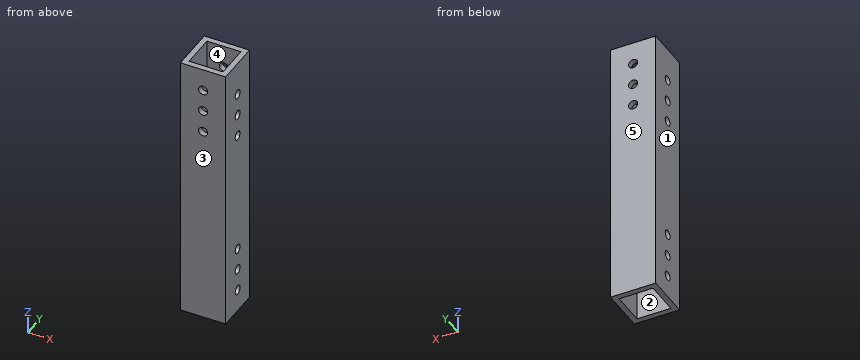
from build123d import *

# Parameters (mm, degrees)
SKETCH3_W              = 25.4
SKETCH3_H              = 25.4
SKETCH3_W_2            = 19.05
SKETCH3_H_2            = 19.05
BOSS_EXTRUDE1_DEPTH    = 152.4
F_10_CLEARANCE_HOLE1_D = 5.1054
F_10_CLEARANCE_HOLE2_D = 5.1054
F_10_CLEARANCE_HOLE3_D = 5.1054


with BuildPart() as part:
    # Sketch3 → Boss-Extrude1 (new body)
    with BuildSketch(Plane.XY):
        with Locations((-12.7, 12.7)):
            Rectangle(SKETCH3_W, SKETCH3_H)
        with Locations((-12.7, 12.7)):
            Rectangle(SKETCH3_W_2, SKETCH3_H_2, mode=Mode.SUBTRACT)
    extrude(amount=BOSS_EXTRUDE1_DEPTH)

    # #10 Clearance Hole1 (through all)
    with Locations(Plane(origin=(0, 25.4, 0), x_dir=(1, 0, 0), z_dir=(0, 1, 0))):
        with Locations((-12.7, -139.7), (-12.7, -127), (-12.7, -114.3)):
            Hole(F_10_CLEARANCE_HOLE1_D / 2)

    # #10 Clearance Hole2 (through all)
    with Locations(Plane.ZY.offset(25.4)):
        with Locations((133.35, 12.7), (120.65, 12.7), (107.95, 12.7)):
            Hole(F_10_CLEARANCE_HOLE2_D / 2)

    # #10 Clearance Hole3 (through all)
    with Locations(Plane(origin=(0, 0, 0), x_dir=(0, 0, -1), z_dir=(1, 0, 0))):
        with Locations((-12.7, 12.7), (-25.4, 12.7), (-38.1, 12.7)):
            Hole(F_10_CLEARANCE_HOLE3_D / 2)


solid = part.part
Verification items for the finished model (mm, model axes). Face numbers are marked on the shaded views. A direction names the side the tool comes from. Coordinates: 2 decimals unless noted, no trailing zeros. Loops run counter-clockwise (first coordinate to the right, second up) from the corner with the lowest first, then second, coordinate; pieces in that order, holes last. Notation, with made-up numbers: M 25.25,32 L 33.25,32 A17 cw 33.25,39 Z; hole C -5.5,41 d1. An arc over 180 degrees is marked long. One line per item, written item: value.
1. Section check B-B on y = 19. Record the cut outline in (x, z) (3 decimals), plus the area to 3 significant figures.
Answers follow:
outline: M -25.4,0 L -22.225,0 L -22.225,152.4 L -25.4,152.4 Z; M -3.175,0 L 0,0 L 0,152.4 L -3.175,152.4 Z
area: 968 mm^2
2. Section check C-C on x = -6. Record the cut outline in (y, z) (3 decimals), plus the area to 3 significant figures.
Answers follow:
outline: M 0,0 L 3.175,0 L 3.175,152.4 L 0,152.4 Z; M 22.225,0 L 25.4,0 L 25.4,152.4 L 22.225,152.4 Z
area: 968 mm^2
3. Section check A-A on z = 12.7. Record the cut outline in (x, y) (3 decimals).
Answers follow:
outline: M -25.4,0 L 0,0 L 0,10.147 L -3.175,10.147 L -3.175,3.175 L -22.225,3.175 L -22.225,10.147 L -25.4,10.147 Z; M -25.4,15.253 L -22.225,15.253 L -22.225,22.225 L -3.175,22.225 L -3.175,15.253 L 0,15.253 L 0,25.4 L -25.4,25.4 Z
4. Set-up check for the marked faces 4 and 5: record each of +Z, -Z, +X, -X, +Y, -Y from which the full face is reachable in a straight line by a thin tool's end or side.
Answers follow:
face 4: +Z, -Z
face 5: +Z, -Z, +X, -X, +Y
5. Material ranges on line 1 along Z through (x, y) = (-12.7, 22.95); line 2 along X through (y, z) = (6.75, 144) (3 decimals); line 3 along Y through (x, z) = (-3.25, 25) (3 decimals), recorded low to high. Write a range as from..to.
Answers follow:
line 1: 0..111.75, 116.85..124.45, 129.55..137.15, 142.25..152.4
line 2: -25.4..-22.225, -3.175..0
line 3: 0..3.175, 22.225..25.4
6. Mould release check, pull along X, two halves, no side actions. Record for the marked faces 1, 2 and 3: pulls with the +X half, pulls with the -X half, needs draft (parallel to the pull), parting line crosses it, or undercut.
Answers follow:
face 1: pulls with the -X half
face 2: undercut
face 3: needs draft
7. Section check D-D on z = 90. Record the cut outline in (x, y) (3 decimals).
Answers follow:
outline: M -25.4,0 L 0,0 L 0,25.4 L -25.4,25.4 Z; hole M -22.225,3.175 L -3.175,3.175 L -3.175,22.225 L -22.225,22.225 Z
